Design review of the part shown in the three views and the two pictorial views. Dimensions are in mm from the part's minimum x, y and z. Coordinates: 2 decimals unless noted, no trailing zeros. Loops run counter-clockwise (first coordinate to the right, second up) from the corner with the lowest first, then second, coordinate; pieces in that order, holes last. Notation, with made-up numbers: M -23,-21 L -18,-21 A28 cw -18,17 Z; hole C -4.75,43 d8. An arc over 180 degrees is marked long. Use one line per item in the form item = value.
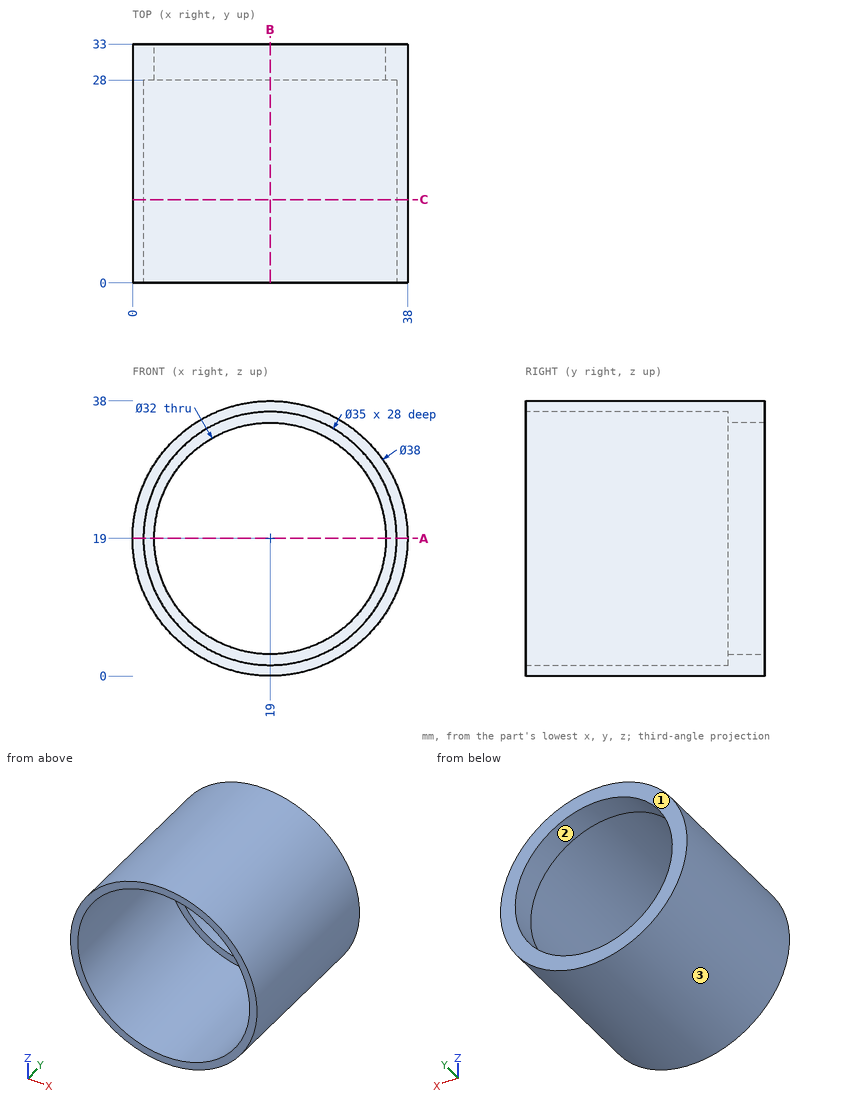
1. Wall thickness on line 1 along X through (y, z) = (30, 19); line 2 along Z through (x, y) = (32, 28.5); line 3 along Y through (x, z) = (24, 2.5): over which ranges is each line inside the solid? List them lowest first. Write a range as from..to.
Response values:
line_1 = 0..3, 35..38
line_2 = 5.14..9.67, 28.33..32.86
line_3 = 28..33
2. Add section A-A (z = 19). State the section outline as (x, y) points, then the cut area to 3 significant figures.
Response values:
outline = M 0,0 L 1.5,0 L 1.5,28 L 3,28 L 3,33 L 0,33 Z; M 35,28 L 36.5,28 L 36.5,0 L 38,0 L 38,33 L 35,33 Z
area = 114 mm^2
3. Insertion check: P1, Ø4, axis at y = 4.5, z = 7, coming from the -X side; P2, Ø1, axis at y = 26.5, z = 16.5, coming from the +X side; P3, Ø1.5, axis at x = 5.5, z = 34, coming from the -Y side; P4, Ø1.5, axis at y = 17, z = 7, coming from the -X side. Each pin has a flat end and moves straight along its axis. Give the tip position at first contact, or say it passes through.
Response values:
P1 = 2.84
P2 = 37.89
P3 = through
P4 = 3.69
4. The part is to be moulded in two halves that separate along Z. For the marked faces 1, 2 and 3, say which applies: pulls with the +Z half, pulls with the -Z half, needs draft (parallel to the pull), parting line crosses it, or undercut.
Response values:
face_1 = needs draft
face_2 = undercut
face_3 = parting line crosses it
5. Add section B-B (x = 19). State the section outline as (y, z) points.
Response values:
outline = M 0,0 L 33,0 L 33,3 L 28,3 L 28,1.5 L 0,1.5 Z; M 0,36.5 L 28,36.5 L 28,35 L 33,35 L 33,38 L 0,38 Z
6. Add section C-C (y = 11.5). State the section outline as (x, z) points, then the cut area to 3 significant figures.
Response values:
outline = C 19,19 d38; hole C 19,19 d35
area = 172 mm^2
